Here's how the part is built. I have some questions about the finished solid (model axes, mm). Round coordinates to 2 decimals unless told otherwise and drop trailing zeros. Loops run counter-clockwise (first coordinate to the right, second up) from the corner with the lowest first, then second, coordinate; pieces in that order, holes last. Notation, with made-up numbers: M 13.5,45 L 20.5,45 A16 cw 20.5,72 Z; hole C 52.5,54 d1. An arc over 180 degrees is marked long. Use a Markdown table: item, result.
Autodesk Inventor part; units mm, degrees
ref_plane "YZ Plane" through (0, 0, 0) normal (1, 0, 0) x (0, 1, 0)
ref_plane "XZ Plane" through (0, 0, 0) normal (0, 1, 0) x (-1, 0, 0)
ref_plane "XY Plane" through (0, 0, 0) normal (0, 0, 1) x (1, 0, 0)
sketch "Sketch1" plane through (0, 0, 0) normal (0, 0, 1) x (1, 0, 0)
  line L0 (0.5, 0) -> (20.5, 0)
  line L1 (21, 0.5) -> (21, 20.5)
  line L2 (20.5, 21) -> (0.5, 21)
  line L3 (0, 20.5) -> (0, 0.5)
  line L4 (0, 20.5) -> (0, 20)
  line L5 (1, 21) -> (0.5, 21)
  line L6 (0, 1) -> (0, 0.5)
  line L7 (0.5, 0) -> (1, 0)
  line L8 (21, 20) -> (21, 20.5)
  line L9 (20.5, 21) -> (20, 21)
  line L10 (20, 0) -> (20.5, 0)
  line L11 (21, 0.5) -> (21, 1)
  arc A0 (0.5, 21) -> (0, 20.5) centre (0.5, 20.5) ccw
  arc A1 (21, 20.5) -> (20.5, 21) centre (20.5, 20.5) ccw
  arc A2 (20.5, 0) -> (21, 0.5) centre (20.5, 0.5) ccw
  arc A3 (0, 0.5) -> (0.5, 0) centre (0.5, 0.5) ccw
  line L12 (0, 21) -> (0, 19.5)
  line L13 (0, 19.5) -> (3, 19.5)
  line L14 (21, 21) -> (21, 19.5)
  line L15 (21, 19.5) -> (18, 19.5)
  line L16 (3, 19.5) -> (3, 18)
  line L17 (18, 19.5) -> (18, 18)
  circle A4 centre (3, 18) radius 1.5
  circle A5 centre (18, 18) radius 1.5
  point P0 (0, 0)
  dimension "d4" = 1.5
  dimension "d5" = 3
  dimension "d6" = 1.5
  dimension "d7" = 3
  dimension "d8" = 1.5
  dimension "d9" = 1.5
extrude "Extrusion1" add sketch "Sketch1" along normal blind 1
sketch "Sketch2" plane through (0, 0, 1) normal (0, 0, 1) x (1, 0, 0)
  line L0 (20.5, 21) -> (0.5, 21)
  circle A0 centre (18, 18) radius 1.5
  circle A1 centre (3, 18) radius 1.5
  line L1 (20.5, 21) -> (0.5, 21)
  arc A2 (0.5, 21) -> (0, 20.5) centre (0.5, 20.5) ccw
  line L2 (0, 20.5) -> (0, 0.5)
  arc A3 (0, 0.5) -> (0.5, 0) centre (0.5, 0.5) ccw
  line L3 (0.5, 0) -> (20.5, 0)
  arc A4 (20.5, 0) -> (21, 0.5) centre (20.5, 0.5) ccw
  line L4 (21, 0.5) -> (21, 20.5)
  arc A5 (21, 20.5) -> (20.5, 21) centre (20.5, 20.5) ccw
  point P0 (0, 0)
properties part number "RGBsensor"
1. Imagine slicing it at C-C, the plane z = 0.35. Write out the boundary of the cut face in (x, y), then the cut area to 3 significant figures.
Answer sheet:
| item | result |
|---|---|
| outline | M 0,0.5 A0.5 ccw 0.5,0 L 20.5,0 A0.5 ccw 21,0.5 L 21,20.5 A0.5 ccw 20.5,21 L 0.5,21 A0.5 ccw 0,20.5 Z; hole C 3,18 d3; hole C 18,18 d3 |
| area | 427 mm2 |
2. I need wall thicknesses on probe 1 along X at (y, z) = (18, 0.3); probe 2 along Y at (x, z) = (18, 0.4). Which ranges of each line are inside material? Lowest first, please. Write a range as from..to.
Answer sheet:
| item | result |
|---|---|
| probe 1 | 0..1.5, 4.5..16.5, 19.5..21 |
| probe 2 | 0..16.5, 19.5..21 |
3. Imagine slicing it at A-A, the plane y = 18. Write out the boundary of the cut face in (x, z).
Answer sheet:
| item | result |
|---|---|
| outline | M 0,0 L 1.5,0 L 1.5,1 L 0,1 Z; M 4.5,0 L 16.5,0 L 16.5,1 L 4.5,1 Z; M 19.5,0 L 21,0 L 21,1 L 19.5,1 Z |
4. Imagine slicing it at B-B, the plane x = 3. Write out the boundary of the cut face in (y, z), then the cut area to 3 significant figures.
Answer sheet:
| item | result |
|---|---|
| outline | M 0,0 L 16.5,0 L 16.5,1 L 0,1 Z; M 19.5,0 L 21,0 L 21,1 L 19.5,1 Z |
| area | 18.0 mm2 |
5. We'd pull the mould along Y, two halves only. Please class faces 1 (the face through (2.805, 16.513, 0.493)), 2 (the face through (0, 10.6, 0.5)), 3 (the face through (10.4, 0, 0.5)): +Y half, -Y half, draft (parallel to the pull), parting line (faces both ways), or undercut.
Answer sheet:
| item | result |
|---|---|
| face 1 | undercut |
| face 2 | draft |
| face 3 | -Y half |
